from build123d import *

# Parameters (mm, degrees)
IZIM1_R                     = 1.5
Y_KSEKLIK_EKSTR_ZYON1_DEPTH = 3
KES_EKSTR_ZYON1_DEPTH       = 3


with BuildPart() as part:
    # Çizim1 → Yükseklik-Ekstrüzyon1 (new body)
    with BuildSketch(Plane(origin=(0, 0, 0), x_dir=(1, 0, 0), z_dir=(0, 1, 0))):
        with BuildLine():
            Line((-17.5, 100), (17.5, 100))
            Line((17.5, 100), (17.5, 75.773502692))
            ThreePointArc((17.5, 75.773502692), (18.839745962, 70.773502692), (22.5, 67.113248654))
            Line((22.5, 67.113248654), (46.871778265, 53.042195912))
            ThreePointArc((46.871778265, 53.042195912), (51.871778265, 51.70244995), (56.871778265, 53.042195912))
            Line((56.871778265, 53.042195912), (77.852540378, 65.155444566))
            Line((77.852540378, 65.155444566), (95.352540378, 34.844555434))
            Line((95.352540378, 34.844555434), (74.371778265, 22.73130678))
            ThreePointArc((74.371778265, 22.73130678), (70.711524227, 19.071052742), (69.371778265, 14.071052742))
            Line((69.371778265, 14.071052742), (69.371778265, -14.071052742))
            ThreePointArc((69.371778265, -14.071052742), (70.711524227, -19.071052742), (74.371778265, -22.73130678))
            Line((74.371778265, -22.73130678), (95.352540378, -34.844555434))
            Line((95.352540378, -34.844555434), (77.852540378, -65.155444566))
            Line((77.852540378, -65.155444566), (56.871778265, -53.042195912))
            ThreePointArc((56.871778265, -53.042195912), (51.871778265, -51.70244995), (46.871778265, -53.042195912))
            Line((46.871778265, -53.042195912), (22.5, -67.113248654))
            ThreePointArc((22.5, -67.113248654), (18.839745962, -70.773502692), (17.5, -75.773502692))
            Line((17.5, -75.773502692), (17.5, -100))
            Line((17.5, -100), (-17.5, -100))
            Line((-17.5, -100), (-17.5, -75.773502692))
            ThreePointArc((-17.5, -75.773502692), (-18.839745962, -70.773502692), (-22.5, -67.113248654))
            Line((-22.5, -67.113248654), (-46.871778265, -53.042195912))
            ThreePointArc((-46.871778265, -53.042195912), (-51.871778265, -51.70244995), (-56.871778265, -53.042195912))
            Line((-56.871778265, -53.042195912), (-77.852540378, -65.155444566))
            Line((-77.852540378, -65.155444566), (-95.352540378, -34.844555434))
            Line((-95.352540378, -34.844555434), (-74.371778265, -22.73130678))
            ThreePointArc((-74.371778265, -22.73130678), (-70.711524227, -19.071052742), (-69.371778265, -14.071052742))
            Line((-69.371778265, -14.071052742), (-69.371778265, 14.071052742))
            ThreePointArc((-69.371778265, 14.071052742), (-70.711524227, 19.071052742), (-74.371778265, 22.73130678))
            Line((-74.371778265, 22.73130678), (-95.352540378, 34.844555434))
            Line((-95.352540378, 34.844555434), (-77.852540378, 65.155444566))
            Line((-77.852540378, 65.155444566), (-56.871778265, 53.042195912))
            ThreePointArc((-56.871778265, 53.042195912), (-51.871778265, 51.70244995), (-46.871778265, 53.042195912))
            Line((-46.871778265, 53.042195912), (-22.5, 67.113248654))
            ThreePointArc((-22.5, 67.113248654), (-18.839745962, 70.773502692), (-17.5, 75.773502692))
            Line((-17.5, 75.773502692), (-17.5, 100))
        make_face()
        with Locations(Location((-12.5, 95, 0), (0, 0, 270))):
            Circle(IZIM1_R, mode=Mode.SUBTRACT)
        with Locations(Location((12.5, 95, 0), (0, 0, 270))):
            Circle(IZIM1_R, mode=Mode.SUBTRACT)
        with Locations(Location((0, 75, 0), (0, 0, 270))):
            Circle(IZIM1_R, mode=Mode.SUBTRACT)
        with Locations(Location((64.951905284, 37.5, 0), (0, 0, 270))):
            Circle(IZIM1_R, mode=Mode.SUBTRACT)
        with Locations(Location((88.52241336, 36.674682453, 0), (0, 0, 270))):
            Circle(IZIM1_R, mode=Mode.SUBTRACT)
        with Locations(Location((76.02241336, 58.325317547, 0), (0, 0, 270))):
            Circle(IZIM1_R, mode=Mode.SUBTRACT)
        with Locations(Location((64.951905284, -37.5, 0), (0, 0, 270))):
            Circle(IZIM1_R, mode=Mode.SUBTRACT)
        with Locations(Location((76.02241336, -58.325317547, 0), (0, 0, 270))):
            Circle(IZIM1_R, mode=Mode.SUBTRACT)
        with Locations(Location((88.52241336, -36.674682453, 0), (0, 0, 270))):
            Circle(IZIM1_R, mode=Mode.SUBTRACT)
        with Locations(Location((0, -75, 0), (0, 0, 270))):
            Circle(IZIM1_R, mode=Mode.SUBTRACT)
        with Locations(Location((-12.5, -95, 0), (0, 0, 270))):
            Circle(IZIM1_R, mode=Mode.SUBTRACT)
        with Locations(Location((12.5, -95, 0), (0, 0, 270))):
            Circle(IZIM1_R, mode=Mode.SUBTRACT)
        with Locations(Location((-64.951905284, -37.5, 0), (0, 0, 270))):
            Circle(IZIM1_R, mode=Mode.SUBTRACT)
        with Locations(Location((-88.52241336, -36.674682453, 0), (0, 0, 270))):
            Circle(IZIM1_R, mode=Mode.SUBTRACT)
        with Locations(Location((-76.02241336, -58.325317547, 0), (0, 0, 270))):
            Circle(IZIM1_R, mode=Mode.SUBTRACT)
        with Locations(Location((-64.951905284, 37.5, 0), (0, 0, 270))):
            Circle(IZIM1_R, mode=Mode.SUBTRACT)
        with Locations(Location((-76.02241336, 58.325317547, 0), (0, 0, 270))):
            Circle(IZIM1_R, mode=Mode.SUBTRACT)
        with Locations(Location((-88.52241336, 36.674682453, 0), (0, 0, 270))):
            Circle(IZIM1_R, mode=Mode.SUBTRACT)
    extrude(amount=Y_KSEKLIK_EKSTR_ZYON1_DEPTH)

    # Çizim3 → Kes-Ekstrüzyon1 (cut)
    with BuildSketch(Plane(origin=(0, 3, 0), x_dir=(1, 0, 0), z_dir=(0, 1, 0))):
        with BuildLine():
            Line((-20, 24.75), (20, 24.75))
            ThreePointArc((20, 24.75), (24.75, 20), (20, 15.25))
            Line((20, 15.25), (-20, 15.25))
            ThreePointArc((-20, 15.25), (-24.75, 20), (-20, 24.75))
        make_face()
        with BuildLine():
            Line((-20, -15.25), (20, -15.25))
            ThreePointArc((20, -15.25), (24.75, -20), (20, -24.75))
            Line((20, -24.75), (-20, -24.75))
            ThreePointArc((-20, -24.75), (-24.75, -20), (-20, -15.25))
        make_face()
    extrude(amount=-KES_EKSTR_ZYON1_DEPTH, mode=Mode.SUBTRACT)


solid = part.part
Geometry check sheet. Reference: the model listing, model coordinates, mm. A direction names the side the tool comes from. Round coordinates to 2 decimals unless told otherwise and drop trailing zeros. Write each loop counter-clockwise with the first axis right and the second up, starting at its lowest first coordinate (ties: lowest second). Pieces come first, ordered by that corner, then holes. Notation, with made-up numbers: (16, 79) -> (23, 79) arc R34 ccw to (23, 116) -> close; hole circle Ø4 at (-29, 47). An arc over 180 degrees is marked (long way). One line per item, written item: value. Start each with the question number.
(1) Cross-section at C-C, the plane y = 0.45. Give the number of separate pieces and of enclosed holes in the cut face, and give its area (3 significant figures).
(2) Cross-section at A-A, the plane z = 20. Record the cut outline in (x, y), and give its area (3 significant figures).
(3) Access from +Z, -Z, +X, -X, +Y, -Y to the whole of each face (thin tool, end or side, straight path). Record for faces 1 (the flat face through (84.715, 1.479, 28.703)), 2 (the flat face through (1, 0, -1)), 3 (the flat face through (67.215, 1.479, -59.014)), 4 (the flat face through (67.509, 1.479, 59.184)), 5 (the cylindrical face through (-24.75, 1.52, 20.1)).
(4) Go/stop test with flat-tipped pins: pin 1 Ø1 at (x, y) = (-25.5, 2) entering from +Z; pin 2 Ø1.5 at (y, z) = (1, -16) entering from +X; pin 3 Ø0.9 at (y, z) = (2, 82) entering from -X. Record where each tip stops, or that it passes through.
(5) Scan lines: line 1 (Z direction, x = 10, y = 2); line 2 (X direction, y = 0.6, z = 37.5); line 3 (Z direction, x = -20.5, y = 1.7). Record each from-to range of solid material in increasing order. Write a range as [from, to].
(6) Cross-section at D-D, the plane z = -30. Record the cut outline in (x, y), and give its area (3 significant figures).
(7) Draft check along Z on faces 6 (the cylindrical face through (-70.748, 1.479, 19.134)), 7 (the flat face through (-67.215, 1.479, 59.014)), 8 (the flat face through (-86.725, 1.479, -49.788)). Enter one of: +Z half, -Z half, draft (parallel to the pull), parting line (faces both ways), or undercut.
(8) Cross-section at B-B, the plane x = -51. Record the cut outline in (y, z), and give its area (3 significant figures).
Answer:
1. separate pieces: 1
1. enclosed holes: 20
1. area: 20,900 mm²
2. outline: (-71.32, 0) -> (-24.75, 0) -> (-24.75, 3) -> (-71.32, 3) -> close; (24.75, 0) -> (71.32, 0) -> (71.32, 3) -> (24.75, 3) -> close
2. area: 279 mm²
3. face 1: +X, +Y, -Y
3. face 2: +Z, -Z, +X, -X, -Y
3. face 3: -Z, +Y, -Y
3. face 4: +Z, +Y, -Y
3. face 5: +Y, -Y
4. pin 1: z = 65.67
4. pin 2: x = 69.74
4. pin 3: x = -17.5
5. line 1: [-100, -24.75], [-15.25, 15.25], [24.75, 100]
5. line 2: [-93.82, -89.77], [-87.27, -66.45], [-63.45, 63.45], [66.45, 87.27], [89.77, 93.82]
5. line 3: [-68.63, -24.72], [-15.28, 15.28], [24.72, 68.63]
6. outline: (-86.96, 0) -> (86.96, 0) -> (86.96, 3) -> (-86.96, 3) -> close
6. area: 522 mm²
7. face 6: undercut
7. face 7: +Z half
7. face 8: -Z half
8. outline: (0, -51.74) -> (3, -51.74) -> (3, 51.74) -> (0, 51.74) -> close
8. area: 310 mm²
